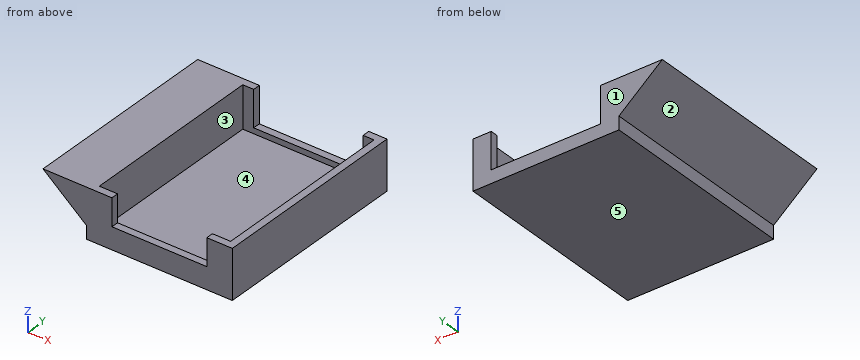
from build123d import *

# Parameters (mm, degrees)
SKETCH_W        = 40
SKETCH_H        = 55
PAD_DEPTH       = 13.5
SKETCH001_W     = 36
SKETCH001_H     = 51
POCKET_DEPTH    = 11.5
SKETCH002_W     = 26
SKETCH002_H     = 7.5
POCKET001_DEPTH = 2
SKETCH003_W     = 30
SKETCH003_H     = 9.959645
POCKET002_DEPTH = 2
PAD001_DEPTH    = 55


with BuildPart() as part:
    # Sketch → Pad (new body)
    with BuildSketch(Plane.XY):
        Rectangle(SKETCH_W, SKETCH_H)
    extrude(amount=PAD_DEPTH)

    # Sketch001 (on Face6 of Pad) → Pocket (cut)
    with BuildSketch(Plane.XY.offset(13.5)):
        Rectangle(SKETCH001_W, SKETCH001_H)
    extrude(amount=-POCKET_DEPTH, mode=Mode.SUBTRACT)

    # Sketch002 (on Face6 of Pocket) → Pocket001 (cut)
    with BuildSketch(Plane.XZ.offset(27.5)):
        with Locations((0, 9.75)):
            Rectangle(SKETCH002_W, SKETCH002_H)
    extrude(amount=-POCKET001_DEPTH, mode=Mode.SUBTRACT)

    # Sketch003 (on Face1 of Pocket001) → Pocket002 (cut)
    with BuildSketch(Plane(origin=(0, 27.5, 0), x_dir=(-1, 0, 0), z_dir=(0, 1, 0))):
        with Locations((0, 8.5201775)):
            Rectangle(SKETCH003_W, SKETCH003_H)
    extrude(amount=-POCKET002_DEPTH, mode=Mode.SUBTRACT)

    # Sketch004 (on Face1 of Pocket002) → Pad001 (join)
    with BuildSketch(Plane(origin=(0, 27.5, 0), x_dir=(-1, 0, 0), z_dir=(0, 1, 0))):
        Polygon((19.9, 13.5), (19.9, 3.5), (31.9, 13.5), align=None)
    extrude(amount=-PAD001_DEPTH)


solid = part.part
The model under review builds one solid part; all positions refer to its coordinate system, in mm. Face numbers are marked on the shaded views. A direction names the side the tool comes from. Round coordinates to 2 decimals unless told otherwise and drop trailing zeros. Write each loop counter-clockwise with the first axis right and the second up, starting at its lowest first coordinate (ties: lowest second). Pieces come first, ordered by that corner, then holes. Notation, with made-up numbers: M 35.5,31.25 L 40.5,31.25 A16 cw 40.5,41.25 Z; hole C -13,82.25 d5. An arc over 180 degrees is marked long. Use a Markdown table: item, result. Add a question column.
Q1. Insertion check: pin 1 (3 mm diameter, centred on x = -6, y = -8.5, fed in from +Z); pin 2 (4 mm diameter, centred on y = 2, z = 1, fed in from -X); pin 3 (1.6 mm diameter, centred on y = 26.5, z = 11, fed in from -X). Each pin has a flat end and moves straight along its axis. Give the tip position at first contact, or say it passes through.
Q2. We need section B-B, the plane y = 17. State the section outline as (x, z) points, plus the area to 3 significant figures.
Q3. We need section A-A, the plane z = 12. State the section outline as (x, y) points, plus the area to 4 significant figures.
Q4. Machinability: for the marked faces 4 and 5, which of the approach directions +Z, -Z, +X, -X, +Y, -Y give a long, thin tool a straight path to every point of the face, cutting with its end or side? Answer none if there is none.
Q5. We need section D-D, the plane z = 5. State the section outline as (x, y) points.
Q6. The part is to be moulded in two halves that separate along X. For the marked faces 1, 2 and 3, say which applies: pulls with the +X half, pulls with the -X half, needs draft (parallel to the pull), parting line crosses it, or undercut.
Q7. We need section C-C, the plane x = -2.5. State the section outline as (y, z) points.
Q8. To check wall thickness, follow line 1 (Y direction, x = -10, z = 2.75); line 2 (Z direction, x = -1, y = -15); line 3 (X direction, y = -19, z = 3.5). State the ranges of each line that lie inside material, in increasing order.
Findings below:
| question | item | result |
|---|---|---|
| 1 | pin 1 | stops at z = 2 |
| 1 | pin 2 | stops at x = -20 |
| 1 | pin 3 | stops at x = -29.86 |
| 2 | outline | M -31.9,13.5 L -20,3.58 L -20,0 L 20,0 L 20,13.5 L 18,13.5 L 18,2 L -18,2 L -18,13.5 Z |
| 2 | area | 185 mm² |
| 3 | outline | M -30.1,-27.5 L -13,-27.5 L -13,-25.5 L -18,-25.5 L -18,25.5 L -15,25.5 L -15,27.5 L -30.1,27.5 Z; M 13,-27.5 L 20,-27.5 L 20,27.5 L 15,27.5 L 15,25.5 L 18,25.5 L 18,-25.5 L 13,-25.5 Z |
| 3 | area | 807.5 mm² |
| 4 | face 4 | +Z |
| 4 | face 5 | -Z, +X, -X, +Y, -Y |
| 5 | outline | M -21.7,-27.5 L 20,-27.5 L 20,27.5 L 15,27.5 L 15,25.5 L 18,25.5 L 18,-25.5 L -18,-25.5 L -18,25.5 L -15,25.5 L -15,27.5 L -21.7,27.5 Z |
| 6 | face 1 | needs draft |
| 6 | face 2 | pulls with the -X half |
| 6 | face 3 | undercut |
| 7 | outline | M -27.5,0 L 27.5,0 L 27.5,3.54 L 25.5,3.54 L 25.5,2 L -25.5,2 L -25.5,6 L -27.5,6 Z |
| 8 | line 1 | y = -27.5 to -25.5, 25.5 to 27.5 |
| 8 | line 2 | z = 0 to 2 |
| 8 | line 3 | x = -20 to -18, 18 to 20 |
